Work out the finished part from the listing and answer in its coordinate system (mm). Face numbers are marked on the shaded views. A direction names the side the tool comes from. Give positions to 0.01 mm unless a question says otherwise; leave off trailing zeros. Loops run counter-clockwise (first coordinate to the right, second up) from the corner with the lowest first, then second, coordinate; pieces in that order, holes last. Notation, with made-up numbers: (-16, -7.5) - (22, -7.5) arc R37 ccw to (22, 31.5) - close; hole circle Ø4 at (4, 72). An arc over 180 degrees is marked (long way). Use CSV: the item, a comma, the result in double quotes.
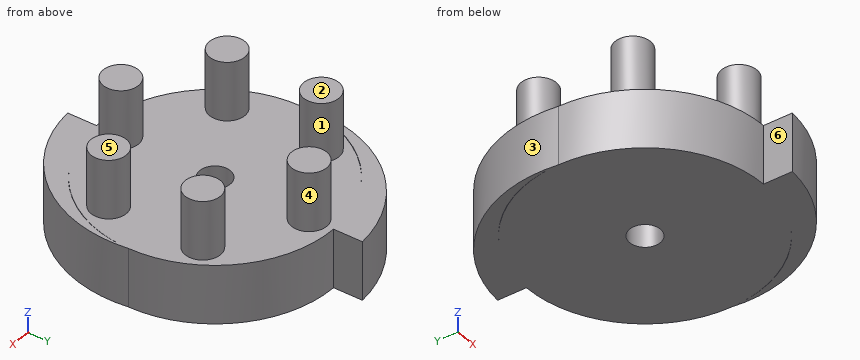
from build123d import *

# Parameters (mm, degrees)
F0_R     = 25.4
F1_DEPTH = 12.7
F3_DEPTH = 12.7
F4_R     = 3.81
F5_DEPTH = 12.7
F6_R     = 3.302
F7_DEPTH = 12.7


with BuildPart() as f1:
    # F0 (on Top) → F1 (new body)
    with BuildSketch(Plane.XY):
        Circle(F0_R)
    extrude(amount=-F1_DEPTH)

    # F2 (on Top) → F3 (join)
    with BuildSketch(Plane.XY):
        with BuildLine():
            ThreePointArc((-25.388571, 0), (-18.019038, 17.965669), (0, 25.203731))
            Line((0, 25.203731), (0, 31.581391))
            ThreePointArc((0, 31.581391), (-19.572424, 21.320095), (-25.388571, 0))
        make_face()
        with BuildLine():
            Line((0, -25.203731), (0, -31.581391))
            ThreePointArc((0, -31.581391), (19.572424, -21.320095), (25.388571, 0))
            ThreePointArc((25.388571, 0), (18.019038, -17.965669), (0, -25.203731))
        make_face()
    extrude(amount=-F3_DEPTH)

    # F4 (on Top) → F5 (join)
    with BuildSketch(Plane.XY):
        with Locations((-17.467251, 10.084722)):
            Circle(F4_R)
        with Locations((0, 20.169444)):
            Circle(F4_R)
        with Locations((17.467251, 10.084722)):
            Circle(F4_R)
        with Locations((17.467251, -10.084722)):
            Circle(F4_R)
        with Locations((0, -20.169444)):
            Circle(F4_R)
        with Locations((-17.467251, -10.084722)):
            Circle(F4_R)
    extrude(amount=F5_DEPTH)

    # F6 (on Top) → F7 (cut)
    with BuildSketch(Plane.XY):
        Circle(F6_R)
    extrude(amount=-F7_DEPTH, mode=Mode.SUBTRACT)


solid = f1.part
Item 1: Find the intervals of material crossed by line 1 (X direction, y = 0.5, z = -9.5); line 2 (Z direction, x = 21.5, y = -12.5); line 3 (X direction, y = 8, z = 6), in increasing order.
Determined:
line 1,"x = -25.46 to -3.26, 3.26 to 25.4"
line 2,"z = -12.7 to 0"
line 3,"x = -20.66 to -14.28, 14.28 to 20.66"
Item 2: A cutting plane is placed at B-B on x = 22. Determine the outline of the cut face in (y, z), and give its area (3 significant figures).
Determined:
outline,"(-17.77, -12.7) - (-12.82, -12.7) - (-12.82, 0) - (-17.77, 0) - close; (-12.69, -12.7) - (12.69, -12.7) - (12.69, 0) - (-12.69, 0) - close"
area,"385 mm²"
Item 3: A cutting plane is placed at C-C on z = -1. Determine the outline of the cut face in (x, y).
Determined:
outline,"(-25.4, 0.08) arc R25.4 ccw to (0, -25.4) - (0, -31.58) arc R27.67 ccw to (25.4, -0.08) arc R25.4 ccw to (0, 25.4) - (0, 31.58) arc R27.67 ccw to start; hole (-25.37, 1.13) arc R25.4 cw to (-13.26, 21.66) arc R24.95 ccw to start; hole circle Ø6.6 at (0, 0); hole (13.26, -21.66) arc R24.95 ccw to (25.37, -1.13) arc R25.4 cw to start"
Item 4: A cutting plane is placed at A-A on y = 4. Determine the outline of the cut face in (x, z).
Determined:
outline,"(-25.68, -12.7) - (-25.11, -12.7) - (-25.11, 0) - (-25.68, 0) - close; (-25.08, -12.7) - (25.08, -12.7) - (25.08, 0) - (-25.08, 0) - close"
Item 5: The mould has two halves that part along X. Classify the marked faces 1, 2 and 3: pulls with the +X half, pulls with the -X half, needs draft (parallel to the pull), parting line crosses it, or undercut.
Determined:
face 1,"undercut"
face 2,"needs draft"
face 3,"pulls with the -X half"
Item 6: For the marked faces 4, 5 and 6, determine the directions among +Z, -Z, +X, -X, +Y, -Y from which every point of the face is accessible in a straight line to the end or side of a thin tool.
Determined:
face 4,"+Z"
face 5,"+Z, +X, -X, +Y, -Y"
face 6,"+Z, -Z, -X, -Y"
Item 7: Given P1, Ø1.9, axis at y = -29.5, z = -4, coming from the -X side; P2, Ø2, axis at y = 6, z = -8, coming from the -X side; P3, Ø2, axis at x = 19.5, z = 3, coming from the +Y side; P4, Ø12, axis at x = -10.5, y = 14.5, coming from the +Z side, each flat-ended and moving along its own axis, determine where each tip first touches the part or whether it passes through.
Determined:
P1,"stops at x = 0"
P2,"stops at x = -25.66"
P3,"stops at y = 13.75"
P4,"stops at z = 12.7"
